Verification items for the finished model (mm, model axes). Give positions to 0.01 mm unless a question says otherwise; leave off trailing zeros. Order: outer loops, then holes, each group sorted by start corner. A loop starts at its lowest first (then second) coordinate and runs counter-clockwise, first axis right, second up. Notation, with made-up numbers: (35, 58) -> (49, 58) arc R25 cw to (49, 74) -> close; hole circle Ø9 at (-19.75, 51.25). An arc over 180 degrees is marked (long way). Return JSON: item names as keys, results as strings. Group by question number.
(1) Thickness scan on line 1 along Y through (x, z) = (240, 1.95); line 2 along Y through (x, z) = (10, 2.75); line 3 along X through (y, z) = (-53.5, 2.75). Record the ranges inside material, lowest first.
(2) Depth check by flat-ended pin: pin 1 Ø1.5 at (x, z) = (231.5, 2.5) entering from -Y; pin 2 Ø1.5 at (y, z) = (-78, 2.5) entering from +X. Enter the tip coordinate at first touch or a pass-through.
(3) Cross-section at C-C on z = 3.35. Enter the section's corners in (x, y), then the cut area to 3 significant figures.
(4) Cross-section at B-B on x = 240. Enter the section's corners in (y, z).
(5) Cross-section at A-A on y = -5. Enter the section's corners in (x, z), then the cut area to 3 significant figures.
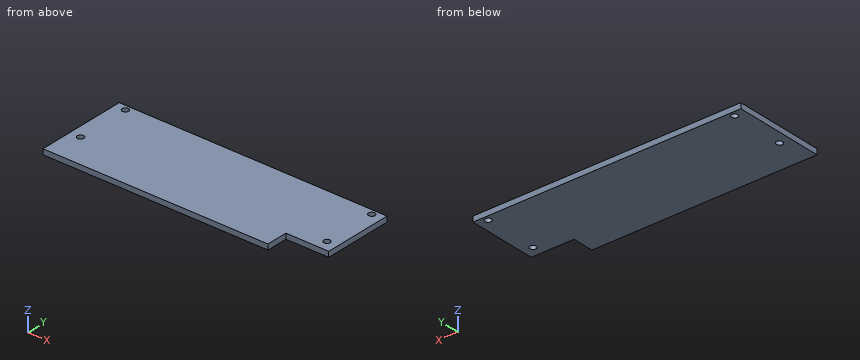
from build123d import *

# Parameters (mm, degrees)
ESQUISSE1_W             = 250
ESQUISSE1_H             = 85
ESQUISSE1_R             = 3
BOSS_EXTRU_1_DEPTH      = 5
ESQUISSE2_W             = 40
ESQUISSE2_H             = 20
ENL_V_MAT_EXTRU_1_DEPTH = 10


with BuildPart() as part:
    # Esquisse1 → Boss.-Extru.1 (new body)
    with BuildSketch(Plane.XY):
        with Locations((125, -42.5)):
            Rectangle(ESQUISSE1_W, ESQUISSE1_H)
        with Locations((10, -5)):
            Circle(ESQUISSE1_R, mode=Mode.SUBTRACT)
        with Locations((10, -55)):
            Circle(ESQUISSE1_R, mode=Mode.SUBTRACT)
        with Locations(Location((240, -55, 0), (0, 0, 180))):
            Circle(ESQUISSE1_R, mode=Mode.SUBTRACT)
        with Locations(Location((240, -5, 0), (0, 0, 180))):
            Circle(ESQUISSE1_R, mode=Mode.SUBTRACT)
    extrude(amount=BOSS_EXTRU_1_DEPTH)

    # Esquisse2 → Enlèv. mat.-Extru.1 (cut)
    with BuildSketch(Plane(origin=(0, 0, 0), x_dir=(-1, 0, 0), z_dir=(0, 0, -1))):
        with Locations((-230, -75)):
            Rectangle(ESQUISSE2_W, ESQUISSE2_H)
    extrude(amount=-ENL_V_MAT_EXTRU_1_DEPTH, mode=Mode.SUBTRACT)


solid = part.part
Verdict:
{
 "1": {"line 1": "-65 to -58, -52 to -8, -2 to 0", "line 2": "-85 to -58, -52 to -8, -2 to 0", "line 3": "0 to 7.4, 12.6 to 237.4, 242.6 to 250"},
 "2": {"pin 1": "y = -65", "pin 2": "x = 210"},
 "3": {"outline": "(0, -85) -> (210, -85) -> (210, -65) -> (250, -65) -> (250, 0) -> (0, 0) -> close; hole circle Ø6 at (10, -55); hole circle Ø6 at (10, -5); hole circle Ø6 at (240, -55); hole circle Ø6 at (240, -5)", "area": "20,300 mm²"},
 "4": {"outline": "(-65, 0) -> (-58, 0) -> (-58, 5) -> (-65, 5) -> close; (-52, 0) -> (-8, 0) -> (-8, 5) -> (-52, 5) -> close; (-2, 0) -> (0, 0) -> (0, 5) -> (-2, 5) -> close"},
 "5": {"outline": "(0, 0) -> (7, 0) -> (7, 5) -> (0, 5) -> close; (13, 0) -> (237, 0) -> (237, 5) -> (13, 5) -> close; (243, 0) -> (250, 0) -> (250, 5) -> (243, 5) -> close", "area": "1,190 mm²"}
}
